The listing builds one solid part. Answer for the finished solid, in the listing's coordinates (mm). Face numbers are marked on the shaded views. A direction names the side the tool comes from. Give positions to 0.01 mm unless a question says otherwise; leave off trailing zeros.
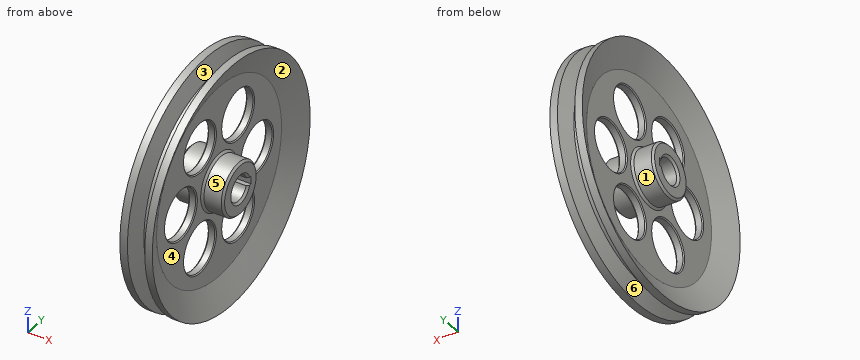
```python
from build123d import *

# Parameters (mm, degrees)
WYTNIJ_WYCI_GNI_CIE1_REACH       = 178.918
SFAZOWANIE2_SIZE                 = 2
SFAZOWANIE3_SIZE                 = 2
WYTNIJ_WYCI_GNI_CIE2_REACH       = 174.166
SZKIC3_R                         = 24
SFAZOWANIE4_SIZE                 = 1
SZYK_KO_OWY2_COUNT               = 6
SFAZOWANIE4_OF_SZYK_KO_OWY2_SIZE = 1


with BuildPart() as part:
    # Szkic1 → Obr_t2 (revolve)
    with BuildSketch(Plane.XY, mode=Mode.PRIVATE) as obr_t2_sk:
        Polygon((-4, 95), (-16, 120), (-8.5, 120), (-2.676476252, 104), (2.676476252, 104), (8.5, 120), (16, 120), (4, 95), (4, 26), (25, 26), (25, 0), (-25, 0), (-25, 26), (-4, 26), align=None)
    revolve(obr_t2_sk.sketch.rotate(Axis((-76.201663435, 0, 0), (1, 0, 0)), 90), axis=Axis((-76.201663435, 0, 0), (1, 0, 0)))

    # Szkic2 → Wytnij-wyci_gni_cie1 (cut, up to next)
    with BuildSketch(Plane.ZY.offset(25), mode=Mode.PRIVATE) as wytnij_wyci_gni_cie1_sk1:
        with BuildLine():
            Line((-4, 16.3), (-4, 11.842719282))
            ThreePointArc((-4, 11.842719282), (0, -12.5), (4, 11.842719282))
            Line((4, 11.842719282), (4, 16.3))
            Line((4, 16.3), (-4, 16.3))
        make_face()
    wytnij_wyci_gni_cie1_tool1 = extrude(wytnij_wyci_gni_cie1_sk1.sketch, amount=-WYTNIJ_WYCI_GNI_CIE1_REACH, mode=Mode.PRIVATE) & part.part
    add(wytnij_wyci_gni_cie1_tool1.solids().sort_by_distance((-25, 0.877795, 0))[0], mode=Mode.SUBTRACT)

    # Sfazowanie2
    sfazowanie2_edges = [part.edges().sort_by_distance(p)[0] for p in [
        (-25, -12.5, 0),
        (25, -12.5, 0),
    ]]
    chamfer(sfazowanie2_edges, length=SFAZOWANIE2_SIZE)

    # Sfazowanie3
    sfazowanie3_edges = [part.edges().sort_by_distance(p)[0] for p in [
        (4, 0, -26),
        (25, 0, -26),
        (-25, 0, -26),
        (-4, 0, -26),
    ]]
    chamfer(sfazowanie3_edges, length=SFAZOWANIE3_SIZE)

    # Szkic3 → Wytnij-wyci_gni_cie2 (cut, up to next)
    with BuildSketch(Plane.ZY.offset(4), mode=Mode.PRIVATE) as wytnij_wyci_gni_cie2_sk1:
        with Locations((0, 58)):
            Circle(SZKIC3_R)
    wytnij_wyci_gni_cie2_tool1 = extrude(wytnij_wyci_gni_cie2_sk1.sketch, amount=-WYTNIJ_WYCI_GNI_CIE2_REACH, mode=Mode.PRIVATE) & part.part
    wytnij_wyci_gni_cie2 = wytnij_wyci_gni_cie2_tool1.solids().sort_by_distance((-4, 58, 0))[0]
    add(wytnij_wyci_gni_cie2, mode=Mode.SUBTRACT)

    # Sfazowanie4
    sfazowanie4_edges = [part.edges().sort_by_distance(p)[0] for p in [
        (-4, 58, -24),
        (4, 58, -24),
    ]]
    chamfer(sfazowanie4_edges, length=SFAZOWANIE4_SIZE)

    # Szyk ko_owy2: Wytnij-wyci_gni_cie2 ×6 about axis
    szyk_ko_owy2_axis = Axis((0, 0, 0), (1, 0, 0))
    for i in range(1, SZYK_KO_OWY2_COUNT):
        add(wytnij_wyci_gni_cie2.rotate(szyk_ko_owy2_axis, i * 360 / SZYK_KO_OWY2_COUNT), mode=Mode.SUBTRACT)

    # Sfazowanie4 of Szyk ko_owy2
    sfazowanie4_of_szyk_ko_owy2_edges = [part.edges().sort_by_distance(p)[0] for p in [
        (-4, 49.784609691, 38.229473419),
        (4, 49.784609691, 38.229473419),
        (-4, -8.215390309, 62.229473419),
        (4, -8.215390309, 62.229473419),
        (-4, -58, 24),
        (4, -58, 24),
        (-4, -49.784609691, -38.229473419),
        (4, -49.784609691, -38.229473419),
        (-4, 8.215390309, -62.229473419),
        (4, 8.215390309, -62.229473419),
    ]]
    chamfer(sfazowanie4_of_szyk_ko_owy2_edges, length=SFAZOWANIE4_OF_SZYK_KO_OWY2_SIZE)


solid = part.part
```
1) For a pull along X with two mould halves and no side action, classify the marked faces 4, 5 and 6 as +X half, -X half, draft (parallel to the pull), parting line (faces both ways), or undercut.
Geometry says:
face 4: +X half
face 5: draft
face 6: undercut
2) Find section A-A (z = -52.5). Count the separate pieces of the cut face and the enclosed holes in it, then the cut area to 3 significant figures.
Geometry says:
separate pieces: 3
enclosed holes: 0
area: 1,240 mm2
3) A tool of negligible diameter and unlimited length cuts with its end or side. For the marked faces 1, 2 and 3, from which of +Z, -Z, +X, -X, +Y, -Y can it reach the whole face along a straight path? Write none if from no direction.
Geometry says:
face 1: -X
face 2: +X
face 3: none
4) Straight lines are drawn through the part: probe 1 along Y at (x, z) = (13, -1); probe 2 along Z at (x, y) = (-12, 2.5); probe 3 along Z at (x, y) = (-0.95, -58). For each, find the intervals that lie inside material, in ascending order.
Geometry says:
probe 1: y = -120 to -113.75, -25.98 to -12.46, 16.3 to 25.98, 113.75 to 120
probe 2: z = -119.97 to -111.64, -25.88 to -12.25, 12.25 to 25.88, 111.64 to 119.97
probe 3: z = -86.32 to -24, 24 to 86.32
5) Given P1, Ø12, axis at x = 18.5, z = -39, coming from the -Y side; P2, Ø4, axis at x = 9.5, y = -12, coming from the -Z side; P3, Ø5, axis at x = -15, y = 36.5, coming from the -Z side, each flat-ended and moving along its own axis, determine where each tip first touches the part or whether it passes through.
Geometry says:
P1: stops at y = -115.22
P2: stops at z = -119.58
P3: stops at z = -115.08
